For this review, use the dimensioned drawing (mm, ordinates from the lowest corner) and the shaded views. A direction names the side the tool comes from. Round coordinates to 2 decimals unless told otherwise and drop trailing zeros. Write each loop counter-clockwise with the first axis right and the second up, starting at its lowest first coordinate (ties: lowest second). Pieces come first, ordered by that corner, then holes. Notation, with made-up numbers: (16.25, 48) - (50.25, 48) arc R12 ccw to (50.25, 67) - close; hole circle Ø10 at (21.25, 80.25). An arc over 180 degrees is marked (long way). Return JSON: item names as keys, results as strings.
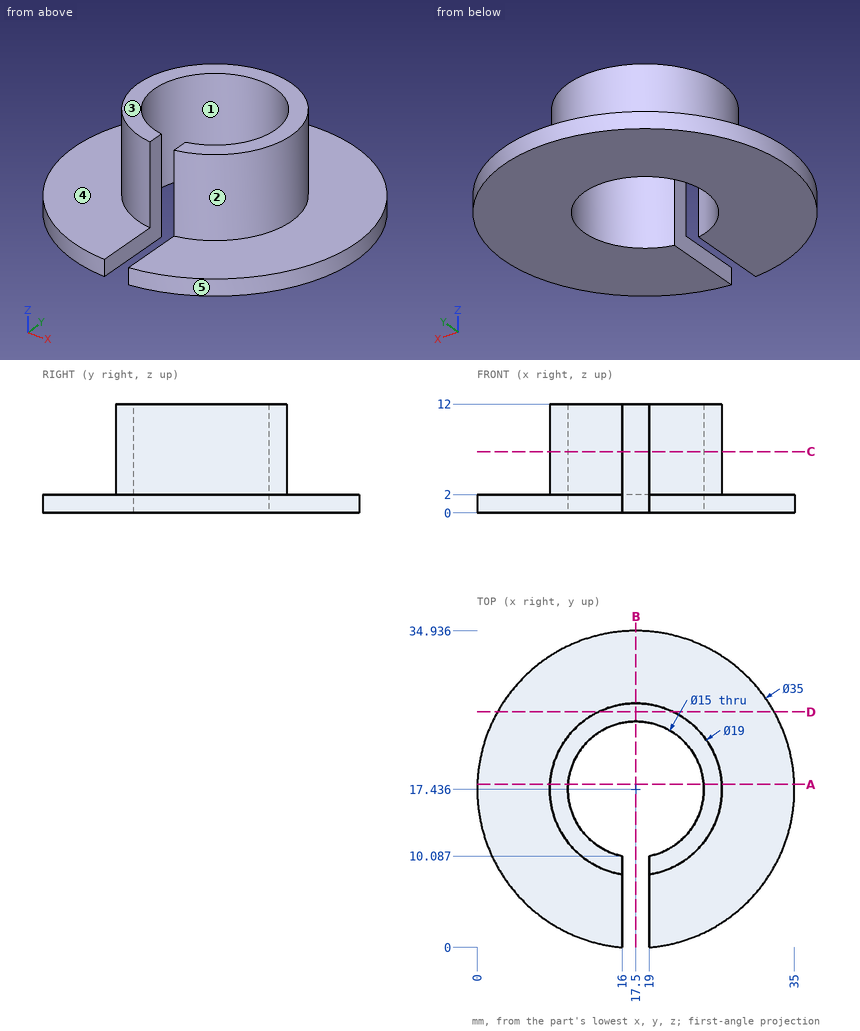
(1) Add section A-A (y = 18). Write out the cut boundary in (x, z).
Filled in:
{"outline": "(0.01, 0) - (10.02, 0) - (10.02, 12) - (8.02, 12) - (8.02, 2) - (0.01, 2) - close; (24.98, 0) - (34.99, 0) - (34.99, 2) - (26.98, 2) - (26.98, 12) - (24.98, 12) - close"}
(2) Add section B-B (x = 17.5). Write out the cut boundary in (y, z) (1 decimal), plus the area to 3 significant figures.
Filled in:
{"outline": "(24.9, 0) - (34.9, 0) - (34.9, 2) - (26.9, 2) - (26.9, 12) - (24.9, 12) - close", "area": "40.0 mm2"}
(3) Mouldability with a two-part tool opening along Y and no side actions: class the marked faces 1, 2 and 3 as released by +Y, released by -Y, zero draft, split by the parting line, or undercut.
Filled in:
{"face 1": "undercut", "face 2": "split by the parting line", "face 3": "zero draft"}
(4) For the marked faces 4 and 5, list the 3-axis set-ups (+Z, -Z, +X, -X, +Y, -Y) from which the entire face can be reached by the end or side of a thin tool; tool diameter is ignored.
Filled in:
{"face 4": "+Z", "face 5": "+Z, -Z"}
(5) Add section D-D (y = 26). Write out the cut boundary in (x, z), plus the area to 3 significant figures.
Filled in:
{"outline": "(2.24, 0) - (32.76, 0) - (32.76, 2) - (21.61, 2) - (21.61, 12) - (13.39, 12) - (13.39, 2) - (2.24, 2) - close", "area": "143 mm2"}
(6) Add section C-C (z = 6.75). Write out the cut boundary in (x, y) (1 decimal), plus the area to 3 significant figures.
Filled in:
{"outline": "(16, 8.1) - (16, 10.1) arc R7.5 cw (long way) to (19, 10.1) - (19, 8.1) arc R9.5 ccw (long way) to start", "area": "101 mm2"}
(7) Wall thickness on line 1 (Y direction, x = 17.5, z = 9.5) (1 decimal); line 2 (Z direction, x = 30, y = 15); line 3 (X direction, y = 22, z = 5): over which ranges is each line inside the solid? List them lowest first.
Filled in:
{"line 1": "y = 24.9 to 26.9", "line 2": "z = 0 to 2", "line 3": "x = 9.17 to 11.55, 23.45 to 25.83"}
(8) Clearance check with flat-ended pins moving along their axes: pin 1 Ø9 at (x, y) = (17.5, 17.44) entering from -Z; pin 2 Ø3 at (x, z) = (26.5, 9.5) entering from +Y (1 decimal); pin 3 Ø1 at (y, z) = (26.5, 6) entering from -X. State where each tip first meets the part, or that it passes through.
Filled in:
{"pin 1": "passes through", "pin 2": "stops at y = 23.3", "pin 3": "stops at x = 13.39"}
